Could you check a few things on this model? Use its own coordinates, in mm. A direction names the side the tool comes from. Coordinates: 2 decimals unless noted, no trailing zeros. Order: outer loops, then holes, each group sorted by start corner. A loop starts at its lowest first (then second) coordinate and runs counter-clockwise, first axis right, second up. Notation, with made-up numbers: M 21.25,-3.75 L 41.25,-3.75 A14 cw 41.25,17.25 Z; hole C 87.5,2.25 d3. An arc over 180 degrees is marked long. One line per question, with ' | ' between items. Start each with the question number.
from build123d import *

# Parameters (mm, degrees)
F0_W     = 25
F0_H     = 3.598708484
F0_H_2   = 2.5
F0_H_3   = 31.6051654611
F0_W_2   = 6
F0_H_4   = 22
F1_DEPTH = 3
F2_DEPTH = 10
F3_START = 10
F3_DEPTH = 3
F4_R     = 4
F5_R     = 3


# Not quite as in the source:
# - a feature names something its author has since deleted; it is built from what else it names


with BuildPart() as f1:
    # F0 (on Top) → F1 (new body)
    with BuildSketch(Plane.XY):
        with Locations((0.1855289564, 2.9724632242)):
            Rectangle(F0_W, F0_H)
        with Locations((0.1855289564, -0.0768910178)):
            Rectangle(F0_W, F0_H_2)
        with Locations((0.1855289564, 20.5744001968)):
            Rectangle(F0_W, F0_H_3)
        with Locations((-6.4080492333, 21.2351317182)):
            Rectangle(F0_W_2, F0_H_4, mode=Mode.SUBTRACT)
        with Locations((6.5919507667, 21.2351317182)):
            Rectangle(F0_W_2, F0_H_4, mode=Mode.SUBTRACT)
    extrude(amount=F1_DEPTH)

    # F0 (on Top) → F2 (join)
    with BuildSketch(Plane.XY):
        with Locations((0.1855289564, -0.0768910178)):
            Rectangle(F0_W, F0_H_2)
    extrude(amount=F2_DEPTH)

    # F0 (on Top) → F3 (join)
    with BuildSketch(Plane.XY.offset(F3_START)):
        with Locations((0.1855289564, 2.9724632242)):
            Rectangle(F0_W, F0_H)
        Polygon((-12.3144710436, -1.3268910178), (-12.3144710436, 1.1731089822), (-12.3144710436, 4.7718174662), (-15.4697376937, 4.7718174662), (-15.4697376937, -5.2281825338), (16.5302623063, -5.2281825338), (16.5302623063, 4.7718174662), (12.6855289564, 4.7718174662), (12.6855289564, 1.1731089822), (12.6855289564, -1.3268910178), align=None)
        with Locations((0.1855289564, -0.0768910178)):
            Rectangle(F0_W, F0_H_2)
    extrude(amount=F3_DEPTH)

    # F4
    f4_edges = [f1.edges().sort_by_distance(p)[0] for p in [
        (16.530262, -5.228183, 11.5),
        (16.530262, 4.771817, 11.5),
        (-15.469738, -5.228183, 11.5),
        (-15.469738, 4.771817, 11.5),
    ]]
    fillet(f4_edges, radius=F4_R)

    # F5
    f5_edges = [f1.edges().sort_by_distance(p)[0] for p in [
        (-12.314471, 36.376983, 1.5),
        (12.685529, 36.376983, 1.5),
    ]]
    fillet(f5_edges, radius=F5_R)


solid = f1.part
(1) For P1, Ø1.5, axis at y = 25, z = 2, coming from the -X side; P2, Ø7.5, axis at x = -2.5, z = 5.5, coming from the +Y side; P3, Ø6, axis at y = 2, z = 2, coming from the +X side; P4, Ø12.5, axis at x = 6, y = 19.5, coming from the +Z side, each with a flat end and sliding along its axis, tell me the tip position at first contact or that it passes through.
(2) Imagine slicing it at B-B, the plane x = 9. Write out the boundary of the cut face in (y, z).
(3) Imagine slicing it at C-C, the plane z = 1.25. Write out the boundary of the cut face in (x, y), plus the area to 3 significant figures.
(4) We'd pull the mould along Y, two halves only. Please class faces 1 (the flat face through (-9.408, 21, 1)), 2 (the flat face through (0, 0, 13)), 3 (the flat face through (0, -1.327, 5)), 4 (the flat face through (-3.408, 21, 1)): +Y half, -Y half, draft (parallel to the pull), parting line (faces both ways), or undercut.
(5) If I drill on line 1 along X through (y, z) = (20, 2); line 2 along X through (y, z) = (6, 1.75); line 3 along Y through (x, z) = (4, 2), over which ranges is the centre line in solid material (lowest first)? Write a range as from..to.
(6) On a 3-axis mill with a long thin cutter (end or side, diameter ignored), from which of +Z, -Z, +X, -X, +Y, -Y can I reach the whole of each face in a straight line? I mean faces 5 (the flat face through (1, 4.772, 11)), 6 (the flat face through (12.686, 11.9, 2.7)), 7 (the flat face through (-12.314, 12.4, 2.7)). Say none if no direction works.
(7) Imagine slicing it at A-A, the plane y = 31.5. Write out the boundary of the cut face in (x, z), plus the area to 3 significant figures.
(8) Imagine slicing it at D-D, the plane z = 12. Write out the boundary of the cut face in (x, y).
Answers:
1) P1: x = -12.31 | P2: y = 36.38 | P3: x = 12.69 | P4: z = 3
2) outline: M -5.23,10 L -1.33,10 L -1.33,0 L 10.24,0 L 10.24,3 L 1.17,3 L 1.17,10 L 4.77,10 L 4.77,13 L -5.23,13 Z; M 32.24,0 L 36.38,0 L 36.38,3 L 32.24,3 Z
3) outline: M -12.31,-1.33 L 12.69,-1.33 L 12.69,33.38 A3 ccw 9.69,36.38 L -9.31,36.38 A3 ccw -12.31,33.38 Z; hole M -9.41,10.24 L -3.41,10.24 L -3.41,32.24 L -9.41,32.24 Z; hole M 3.59,10.24 L 9.59,10.24 L 9.59,32.24 L 3.59,32.24 Z | area: 675 mm²
4) face 1: undercut | face 2: draft | face 3: -Y half | face 4: undercut
5) line 1: -12.31..-9.41, -3.41..3.59, 9.59..12.69 | line 2: -12.31..12.69 | line 3: -1.33..10.24, 32.24..36.38
6) face 5: +Z, +X, -X, +Y | face 6: -Z, +X, +Y, -Y | face 7: -Z, -X, +Y, -Y
7) outline: M -12.31,0 L -9.41,0 L -9.41,3 L -12.31,3 Z; M -3.41,0 L 3.59,0 L 3.59,3 L -3.41,3 Z; M 9.59,0 L 12.69,0 L 12.69,3 L 9.59,3 Z | area: 39.0 mm²
8) outline: M -15.47,-1.23 A4 ccw -11.47,-5.23 L 12.53,-5.23 A4 ccw 16.53,-1.23 L 16.53,0.77 A4 ccw 12.53,4.77 L -11.47,4.77 A4 ccw -15.47,0.77 Z
